Can you work these out from the model? Positions are in its coordinate system, mm. A direction names the side the tool comes from. Coordinates: 2 decimals unless noted, no trailing zeros. Write each loop counter-clockwise with the first axis right and the second up, starting at its lowest first coordinate (ties: lowest second). Pieces come first, ordered by that corner, then holes.
Autodesk Inventor part; units mm, degrees
ref_plane "YZ Plane" through (0, 0, 0) normal (1, 0, 0) x (0, 1, 0)
ref_plane "XZ Plane" through (0, 0, 0) normal (0, 1, 0) x (-1, 0, 0)
ref_plane "XY Plane" through (0, 0, 0) normal (0, 0, 1) x (1, 0, 0)
sketch "Boceto1" plane through (0, 0, 0) normal (0, 1, 0) x (-1, 0, 0)
  line L0 (-40, 8) -> (40, 8)
  line L1 (40, 8) -> (40, -8)
  line L2 (40, -8) -> (-40, -8)
  line L3 (-40, -8) -> (-40, 8)
  line L4 (-40, 8) -> (40, -8) construction
  line L5 (40, 8) -> (-40, -8) construction
  circle A0 centre (-16.7, 4) radius 2.7
  circle A1 centre (-16.7, -4) radius 2.7
  circle A2 centre (16.7, 4) radius 2.7
  circle A3 centre (16.7, -4) radius 2.7
  line L6 (19.4, 4) -> (14, 4)
  line L7 (14, 4) -> (14, -4)
  line L8 (14, -4) -> (19.4, -4)
  line L9 (19.4, -4) -> (19.4, 4)
  line L10 (-14, 4) -> (-19.4, 4)
  line L11 (-19.4, 4) -> (-19.4, -4)
  line L12 (-19.4, -4) -> (-14, -4)
  line L13 (-14, -4) -> (-14, 4)
  point P0 (0, 0)
  point P1 (16.7, -4)
  point P2 (16.7, 4)
  point P3 (-16.7, -4)
  point P4 (-16.7, 4)
  point P5 (19.4, -4)
  point P6 (-14, -4)
  point P7 (-19.4, -4)
  point P8 (-19.4, 4)
  dimension "d2" = 5.4
  dimension "d0" = 80
  dimension "d1" = 16
  dimension "d3" = 4
  dimension "d4" = 8
  dimension "d5" = 23.3
  dimension "d35" = 23.3
extrude "Extrusión1" add sketch "Boceto1" along normal blind 5
fillet "Empalme2" radius 3 4 edges at (-40, 2.5, 8) (-40, 2.5, -8) (40, 2.5, 8) (40, 2.5, -8)
sketch "Boceto6" plane through (0, 5, 0) normal (0, 1, 0) x (1, 0, 0)
  circle A0 centre (-30, 0) radius 6.125
  circle A1 centre (30, 0) radius 6.125
  point P0 (0, 0)
  dimension "d27" = 12.25
  dimension "d28" = 30
  dimension "d29" = 30
extrude "Extrusión6" cut sketch "Boceto6" against normal through all
sketch "Boceto7" plane through (0, 0, 0) normal (0, -1, 0) x (1, 0, 0)
  circle A0 centre (-30, 0) radius 6.125
  circle A1 centre (30, 0) radius 6.125
  circle A2 centre (-30, 0) radius 3.5
  circle A3 centre (30, 0) radius 3.5
  point P0 (0, 0)
  point P1 (18.5632, -5.9541)
  point P2 (18.5632, 5.9541)
  dimension "d32" = 7
extrude "Extrusión7" add sketch "Boceto7" against normal blind 1
sketch "Boceto9" plane through (0, 5, 0) normal (0, 1, 0) x (1, 0, 0)
  circle A0 centre (-7, 0.0746) radius 2.7
  circle A1 centre (7, 0.0746) radius 2.7
  point P0 (0, 0)
  dimension "d36" = 5.4
  dimension "d39" = 7
  dimension "d40" = 7
extrude "Extrusión8" cut sketch "Boceto9" against normal through all
sketch "Boceto5" plane through (0, 0, 0) normal (0, -1, 0) x (1, 0, 0)
  circle A0 centre (-30, -4.1) radius 1.7
  circle A1 centre (-30, -4.1) radius 2.875
  circle A2 centre (20, -4.1) radius 1.7
  circle A3 centre (20, -4.1) radius 2.875
  line L0 (-33.3198, -4.1) -> (-31.6599, -1.225)
  line L1 (-31.6599, -1.225) -> (-28.3401, -1.225)
  line L2 (-28.3401, -1.225) -> (-26.6802, -4.1)
  line L3 (-26.6802, -4.1) -> (-28.3401, -6.975)
  line L4 (-28.3401, -6.975) -> (-31.6599, -6.975)
  line L5 (-31.6599, -6.975) -> (-33.3198, -4.1)
  line L6 (16.6802, -4.1) -> (18.3401, -1.225)
  line L7 (18.3401, -1.225) -> (21.6599, -1.225)
  line L8 (21.6599, -1.225) -> (23.3198, -4.1)
  line L9 (23.3198, -4.1) -> (21.6599, -6.975)
  line L10 (21.6599, -6.975) -> (18.3401, -6.975)
  line L11 (18.3401, -6.975) -> (16.6802, -4.1)
  point P0 (0, 0)
  dimension "d24" = 5.75
properties part number "Rack support b"
1. If I drill on L1, parallel to X at y = 1.15, z = 2.75; L2, parallel to Z at x = -30, y = 2.1 (3 decimals); L3, parallel to X at y = 3.55, z = 4.5, over which ranges is the centre line in solid material (lowest first)?
2. We'd pull the mould along Z, two halves only. Please class faces 3 (the face through (1, 2, 8)), 4 (the face through (-36.12, 3.03, -0.27)), 5 (the face through (1, 5, 0)): released by +Z, released by -Z, zero draft, split by the parting line, or undercut.
3. If we section it at C-C, the plane x = -16.7: List the corners of the cut face in (y, z) for me, plus the area to 3 significant figures.
4. If we section it at B-B, the plane y = 2.2: List the corners of the cut face in (x, z) for me (3 decimals), plus the area to 3 significant figures.
5. I'm going to push a flat-ended pin straight in: P1, Ø6, axis at x = -30, z = -2.5, coming from the +Y side. Where does the tip first touch, or does it pass through?
6. If we section it at D-D, the plane z = 1: Count the separate pieces of the cut face and the enclosed holes in it, plus the area to 3 significant figures.
7. Which directions (+Z, -Z, +X, -X, +Y, -Y) give clear straight access to the entire face, cutting with the end or side of a thin tool? Please do faces 1 (the face through (16.8, 2.5, 6.7)), 2 (the face through (39.1, 2.54, 7.14)).
8. If we section it at A-A, the plane x = 7: List the corners of the cut face in (y, z) for me.
Answers:
1. L1: x = -40 to -35.47, -24.53 to -19.4, -14 to 14, 19.4 to 24.53, 35.47 to 40
1. L2: z = -8 to -6.125, 6.125 to 8
1. L3: x = -40 to -34.16, -25.84 to -19.35, -14.05 to 14.05, 19.35 to 25.84, 34.16 to 40
2. face 3: released by +Z
2. face 4: undercut
2. face 5: zero draft
3. outline: (0, -8) - (5, -8) - (5, -6.7) - (0, -6.7) - close; (0, 6.7) - (5, 6.7) - (5, 8) - (0, 8) - close
3. area: 13.0 mm2
4. outline: (-40, -5) arc R3 ccw to (-37, -8) - (37, -8) arc R3 ccw to (40, -5) - (40, 5) arc R3 ccw to (37, 8) - (-37, 8) arc R3 ccw to (-40, 5) - close; hole circle Ø12.25 at (-30, 0); hole (-19.4, -4) arc R2.7 ccw to (-14, -4) - (-14, 4) arc R2.7 ccw to (-19.4, 4) - close; hole circle Ø5.4 at (-7, -0.075); hole circle Ø5.4 at (7, -0.075); hole (14, -4) arc R2.7 ccw to (19.4, -4) - (19.4, 4) arc R2.7 ccw to (14, 4) - close; hole circle Ø12.25 at (30, 0)
4. area: 859 mm2
5. P1: stops at y = 1
6. separate pieces: 7
6. enclosed holes: 0
6. area: 186 mm2
7. face 1: +Y, -Y
7. face 2: +Z, +X, +Y, -Y
8. outline: (0, -8) - (5, -8) - (5, -2.77) - (0, -2.77) - close; (0, 2.63) - (5, 2.63) - (5, 8) - (0, 8) - close
